The model under review builds one solid part; all positions refer to its coordinate system, in mm. Give positions to 0.01 mm unless a question says otherwise; leave off trailing zeros. Loops run counter-clockwise (first coordinate to the right, second up) from the corner with the lowest first, then second, coordinate; pieces in that order, holes last. Notation, with made-up numbers: M 86.25,78.5 L 126.25,78.5 A18 cw 126.25,83.5 Z; hole C -32.5,61.5 d5. An arc over 180 degrees is marked long. Write item = value, one per line. Start each with the question number.
1. We need section C-C on x = 83. Give the boundary of the cut face in (y, z).
2. We need section A-A on y = 84. Give the boundary of the cut face in (x, z), then the cut area to 3 significant figures.
3. We need section B-B on x = 51. Give the boundary of the cut face in (y, z).
4. Wall thickness on line 1 along X through (y, z) = (74, 0.45); line 2 along Y through (x, z) = (52.5, 1.35); line 3 along Y through (x, z) = (9.5, 1.3): over which ranges is each line inside the solid? List them lowest first. Write a range as from..to.
5. For pin 1 (0.8 mm diameter, centred on x = 8.5, z = 0.5, fed in from +Y); pin 2 (4 mm diameter, centred on x = 21.39, y = 72.3, fed in from -Z); pin 3 (0.8 mm diameter, centred on x = 104.5, z = 0.5, fed in from +Y); pin 4 (0.5 mm diameter, centred on y = 97.5, z = 0.5, fed in from +X), all flat-tipped, find the tip position at first contact; note any pin that passes through.
6. We need section D-D on z = 0.3. Count the separate pieces of the cut face and the enclosed holes in it, then the cut area to 3 significant figures.
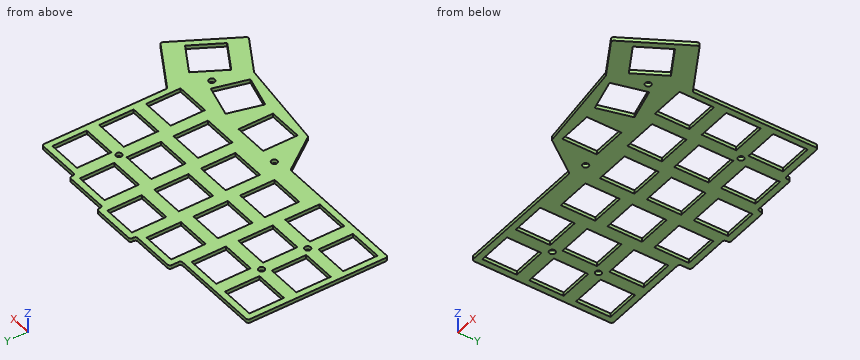
from build123d import *

# Parameters (mm, degrees)
SKETCH2_R           = 1.2
SKETCH2_W           = 13.999999997
SKETCH2_H           = 13.999999996
SKETCH2_W_2         = 13.999999996
SKETCH2_H_2         = 13.999999997
BOSS_EXTRUDE1_DEPTH = 1.5


with BuildPart() as part:
    # Sketch2 → Boss-Extrude1 (new body)
    with BuildSketch(Plane.XY):
        with BuildLine():
            Line((2.396591635, 90.463437274), (2.396591635, 35.387693174))
            ThreePointArc((2.396591635, 35.387693174), (2.678391323, 34.707368546), (3.358715952, 34.425568858))
            Line((3.358715952, 34.425568858), (57.55538108, 34.425568858))
            ThreePointArc((57.55538108, 34.425568858), (57.991412266, 34.32109249), (58.332746845, 34.030353412))
            Line((58.332746845, 34.030353412), (68.6731028, 19.851286658))
            ThreePointArc((68.6731028, 19.851286658), (68.959916761, 19.590522811), (69.326358752, 19.464109602))
            Line((69.326358752, 19.464109602), (106.42211034, 14.638604201))
            ThreePointArc((106.42211034, 14.638604201), (106.606561986, 14.595821202), (106.779062685, 14.517742374))
            Line((106.779062685, 14.517742374), (121.831200494, 5.827386558))
            ThreePointArc((121.831200494, 5.827386558), (122.561278749, 5.731269932), (123.145486752, 6.1795485))
            Line((123.145486752, 6.1795485), (136.883362434, 29.974247168))
            ThreePointArc((136.883362434, 29.974247168), (136.979479059, 30.704325424), (136.531200492, 31.288533426))
            Line((136.531200492, 31.288533426), (116.881014221, 42.63357376))
            ThreePointArc((116.881014221, 42.63357376), (116.52885228, 42.985735701), (116.399952063, 43.466797859))
            Line((116.399952063, 43.466797859), (116.399952063, 92.828345033))
            ThreePointArc((116.399952063, 92.828345033), (116.118152375, 93.508669661), (115.437827746, 93.790469349))
            Line((115.437827746, 93.790469349), (98.360317754, 93.790469349))
            ThreePointArc((98.360317754, 93.790469349), (97.679993126, 94.072269037), (97.398193438, 94.752593666))
            Line((97.398193438, 94.752593666), (97.398193438, 95.213192117))
            ThreePointArc((97.398193438, 95.213192117), (97.11639375, 95.893516746), (96.436069121, 96.175316434))
            Line((96.436069121, 96.175316434), (79.359092742, 96.175316434))
            ThreePointArc((79.359092742, 96.175316434), (78.678768113, 96.457116122), (78.396968425, 97.137440751))
            Line((78.396968425, 97.137440751), (78.396968425, 97.587767164))
            ThreePointArc((78.396968425, 97.587767164), (78.115168737, 98.268091793), (77.434844109, 98.54989148))
            Line((77.434844109, 98.54989148), (60.359092745, 98.54989148))
            ThreePointArc((60.359092745, 98.54989148), (59.678768117, 98.268091793), (59.396968429, 97.587767164))
            Line((59.396968429, 97.587767164), (59.396968429, 97.133171852))
            ThreePointArc((59.396968429, 97.133171852), (59.115168741, 96.452847223), (58.434844112, 96.171047535))
            Line((58.434844112, 96.171047535), (41.357156249, 96.171047535))
            ThreePointArc((41.357156249, 96.171047535), (40.676831621, 95.889247847), (40.395031933, 95.208923218))
            Line((40.395031933, 95.208923218), (40.395031933, 92.387685907))
            ThreePointArc((40.395031933, 92.387685907), (40.113232245, 91.707361278), (39.432907616, 91.42556159))
            Line((39.432907616, 91.42556159), (3.358715952, 91.42556159))
            ThreePointArc((3.358715952, 91.42556159), (2.678391323, 91.143761902), (2.396591635, 90.463437274))
        make_face()
        with Locations((21.387798276, 72.300241098)):
            Circle(SKETCH2_R, mode=Mode.SUBTRACT)
        with Locations((21.387798276, 53.550235091)):
            Circle(SKETCH2_R, mode=Mode.SUBTRACT)
        with Locations((64.637863533, 36.300090173)):
            Circle(SKETCH2_R, mode=Mode.SUBTRACT)
        with Locations((111.137845658, 28.550051811)):
            Circle(SKETCH2_R, mode=Mode.SUBTRACT)
        with Locations((97.387827206, 76.050038887)):
            Circle(SKETCH2_R, mode=Mode.SUBTRACT)
        with Locations((11.896591633, 81.925561592)):
            Rectangle(SKETCH2_W, SKETCH2_H, mode=Mode.SUBTRACT)
        with Locations((78.416585941, 29.017413842)):
            Rectangle(SKETCH2_W_2, SKETCH2_H, mode=Mode.SUBTRACT)
        Polygon((107.952399337, 31.256983985), (104.328932707, 17.734022421), (90.805971142, 21.357489051), (94.429437772, 34.880450616), align=None, mode=Mode.SUBTRACT)
        Polygon((112.075005434, 20.004912386), (119.075005433, 32.129268036), (131.199361083, 25.129268038), (124.199361084, 13.004912388), align=None, mode=Mode.SUBTRACT)
        with Locations((106.899952065, 46.290476615)):
            Rectangle(SKETCH2_W, SKETCH2_H_2, mode=Mode.SUBTRACT)
        with Locations((87.89819344, 48.6753237)):
            Rectangle(SKETCH2_W, SKETCH2_H_2, mode=Mode.SUBTRACT)
        with Locations((68.896968427, 51.049898746)):
            Rectangle(SKETCH2_W_2, SKETCH2_H, mode=Mode.SUBTRACT)
        with Locations((49.895031931, 48.671054801)):
            Rectangle(SKETCH2_W_2, SKETCH2_H_2, mode=Mode.SUBTRACT)
        with Locations((30.894762974, 43.926240308)):
            Rectangle(SKETCH2_W_2, SKETCH2_H, mode=Mode.SUBTRACT)
        with Locations((11.896591633, 43.925568856)):
            Rectangle(SKETCH2_W, SKETCH2_H, mode=Mode.SUBTRACT)
        with Locations((106.899952065, 65.29047661)):
            Rectangle(SKETCH2_W, SKETCH2_H, mode=Mode.SUBTRACT)
        with Locations((87.89819344, 67.675323695)):
            Rectangle(SKETCH2_W, SKETCH2_H_2, mode=Mode.SUBTRACT)
        with Locations((68.896968427, 70.049898741)):
            Rectangle(SKETCH2_W_2, SKETCH2_H, mode=Mode.SUBTRACT)
        with Locations((49.895031931, 67.671054795)):
            Rectangle(SKETCH2_W_2, SKETCH2_H_2, mode=Mode.SUBTRACT)
        with Locations((30.894762974, 62.926240303)):
            Rectangle(SKETCH2_W_2, SKETCH2_H, mode=Mode.SUBTRACT)
        with Locations((11.896591633, 62.925568851)):
            Rectangle(SKETCH2_W, SKETCH2_H, mode=Mode.SUBTRACT)
        with Locations((106.899952065, 84.290469351)):
            Rectangle(SKETCH2_W, SKETCH2_H, mode=Mode.SUBTRACT)
        with Locations((87.89819344, 86.675316436)):
            Rectangle(SKETCH2_W, SKETCH2_H_2, mode=Mode.SUBTRACT)
        with Locations((68.896968427, 89.049891482)):
            Rectangle(SKETCH2_W_2, SKETCH2_H, mode=Mode.SUBTRACT)
        with Locations((49.895031931, 86.671047537)):
            Rectangle(SKETCH2_W_2, SKETCH2_H, mode=Mode.SUBTRACT)
        with Locations((30.894762974, 81.926233044)):
            Rectangle(SKETCH2_W_2, SKETCH2_H, mode=Mode.SUBTRACT)
    extrude(amount=BOSS_EXTRUDE1_DEPTH)


solid = part.part
Final values:
q1.outline = M 17.69,0 L 22.02,0 L 22.02,1.5 L 17.69,1.5 Z; M 36.02,0 L 41.68,0 L 41.68,1.5 L 36.02,1.5 Z; M 55.68,0 L 60.68,0 L 60.68,1.5 L 55.68,1.5 Z; M 74.68,0 L 79.68,0 L 79.68,1.5 L 74.68,1.5 Z; M 93.68,0 L 96.18,0 L 96.18,1.5 L 93.68,1.5 Z
q2.outline = M 2.4,0 L 4.9,0 L 4.9,1.5 L 2.4,1.5 Z; M 18.9,0 L 23.89,0 L 23.89,1.5 L 18.9,1.5 Z; M 37.89,0 L 42.9,0 L 42.9,1.5 L 37.89,1.5 Z; M 56.9,0 L 61.9,0 L 61.9,1.5 L 56.9,1.5 Z; M 75.9,0 L 80.9,0 L 80.9,1.5 L 75.9,1.5 Z; M 94.9,0 L 99.9,0 L 99.9,1.5 L 94.9,1.5 Z; M 113.9,0 L 116.4,0 L 116.4,1.5 L 113.9,1.5 Z
q2.area = 45.0 mm²
q3.outline = M 34.43,0 L 41.67,0 L 41.67,1.5 L 34.43,1.5 Z; M 55.67,0 L 60.67,0 L 60.67,1.5 L 55.67,1.5 Z; M 74.67,0 L 79.67,0 L 79.67,1.5 L 74.67,1.5 Z; M 93.67,0 L 96.17,0 L 96.17,1.5 L 93.67,1.5 Z
q4.line_1 = 2.4..42.9, 56.9..61.9, 75.9..80.9, 94.9..116.4
q4.line_2 = 34.43..41.67, 55.67..60.67, 74.67..79.67, 93.67..96.17
q4.line_3 = 34.43..36.93, 50.93..55.93, 69.93..74.93, 88.93..91.43
q5.pin_1 = 91.43
q5.pin_2 = 0
q5.pin_3 = 93.79
q5.pin_4 = 78.4
q6.separate_pieces = 1
q6.enclosed_holes = 26
q6.area = 4,140 mm²
